Read the model definition and answer for the solid it produces. Units are mm, in the model's axes. A direction names the side the tool comes from. Give positions to 0.01 mm unless a question says otherwise; leave off trailing zeros. Loops run counter-clockwise (first coordinate to the right, second up) from the corner with the lowest first, then second, coordinate; pieces in that order, holes last. Notation, with made-up numbers: (32.25, -12) -> (71.25, -12) arc R23 ccw to (71.25, 24) -> close; hole circle Ø8 at (52, 43). An arc over 180 degrees is marked (long way). Write each question's results on one line, items separated by ' | '. Start each with the question number.
Item 1: Each of these flat-tipped pins is pushed along its axis until it touches: P1, Ø2.5, axis at x = 17.5, z = 3.5, coming from the +Y side; P2, Ø1, axis at x = 23.5, z = 3, coming from the -Y side; P3, Ø4, axis at y = 5, z = 4.5, coming from the +X side. Where does it stop, or does it pass through?
Item 2: Which of the six approach directions +Z, -Z, +X, -X, +Y, -Y give full straight-line access (tool end or side, diameter ignored) to faces 4 (the flat face through (5, 15, 0)), 5 (the flat face through (20, 12.5, 5)), 6 (the flat face through (10, 24, 6))?
Item 3: Section A-A on y = 25 is taken. Write down the section's boundary in (x, z).
Item 4: Section B-B on z = 4.5 is taken. Write down the section's boundary in (x, y), and give its area (3 significant figures).
Item 5: Section D-D on z = 2.5 is taken. Write down the section's boundary in (x, y).
Item 6: Section C-C on x = 3 is taken. Write down the section's boundary in (y, z), and give its area (3 significant figures).
Item 7: Determine the mould class of faces 1 (the conical face through (19.965, 13.768, 7.393)), 2 (the flat face through (0, 15, 5)), 3 (the cylindrical face through (5, 5, 6)) for opening direction X: +X half, -X half, draft (parallel to the pull), parting line (faces both ways), or undercut.
Item 8: Find the intervals of material crossed by line 1 (Y direction, x = 3.25, z = 4.5); line 2 (Y direction, x = 3.5, z = 3.25); line 3 (Z direction, x = 5.25, y = 5), in increasing order.
```python
from build123d import *

# Parameters (mm, degrees)
SKETCH1_W           = 10
SKETCH1_H           = 9
BOSS_EXTRUDE1_DEPTH = 30
SKETCH2_W           = 9
SKETCH2_H           = 5
BOSS_EXTRUDE2_DEPTH = 20
SKETCH3_R           = 1.5
CUT_EXTRUDE1_DEPTH  = 38.161808352


# Read off the part's stored shape, not the designer's step: Cut-Extrude2
with BuildPart() as part:
    # Sketch1 → Boss-Extrude1 (new body)
    with BuildSketch(Plane(origin=(0, 0, 0), x_dir=(1, 0, 0), z_dir=(0, 1, 0))):
        with Locations((5, -4.5)):
            Rectangle(SKETCH1_W, SKETCH1_H)
    extrude(amount=BOSS_EXTRUDE1_DEPTH)

    # Sketch2 → Boss-Extrude2 (add)
    with BuildSketch(Plane(origin=(10, 0, 0), x_dir=(0, 0, -1), z_dir=(1, 0, 0))):
        with Locations((-4.5, 15)):
            Rectangle(SKETCH2_W, SKETCH2_H)
    extrude(amount=BOSS_EXTRUDE2_DEPTH)

    # Sketch3 → Cut-Extrude1 (cut, through all)
    with BuildSketch(Plane(origin=(10, 0, 0), x_dir=(0, 0, -1), z_dir=(1, 0, 0))):
        with Locations((-4.5, 25)):
            Circle(SKETCH3_R)
        with Locations(Location((-4.5, 5, 0), (0, 0, 180))):
            Circle(SKETCH3_R)
    extrude(amount=-CUT_EXTRUDE1_DEPTH, mode=Mode.SUBTRACT)

    # Cut-Extrude2 outline → Cut-Extrude2 (revolve, cut)
    with BuildSketch(Plane(origin=(20, 0, 0), x_dir=(1, 0, 0), z_dir=(0, 0, 1))):
        Polygon((1.718721659, 12.5), (1.5, 15), (1.718721659, 17.5), (0, 17.5), (0, 12.5), align=None)
    cut_extrude2 = revolve(axis=Axis((20, 0, 0), (0, 1, 0)), mode=Mode.SUBTRACT)

    # Mirror1: Cut-Extrude2 across plane
    add(cut_extrude2.mirror(Plane.XY.offset(4.5)), mode=Mode.SUBTRACT)


solid = part.part
```
Findings:
1) P1: y = 17.5 | P2: y = 12.5 | P3: x = 10
2) face 4: -Z, +X, -X, +Y, -Y | face 5: +Z, -Z, +X, -Y | face 6: +Z, -Z, +X, +Y
3) outline: (0, 0) -> (10, 0) -> (10, 3) -> (0, 3) -> close; (0, 6) -> (10, 6) -> (10, 9) -> (0, 9) -> close
4) outline: (0, 0) -> (10, 0) -> (10, 3.5) -> (0, 3.5) -> close; (0, 6.5) -> (10, 6.5) -> (10, 12.5) -> (30, 12.5) -> (30, 17.5) -> (10, 17.5) -> (10, 23.5) -> (0, 23.5) -> close; (0, 26.5) -> (10, 26.5) -> (10, 30) -> (0, 30) -> close | area: 340 mm2
5) outline: (0, 0) -> (10, 0) -> (10, 12.5) -> (30, 12.5) -> (30, 17.5) -> (10, 17.5) -> (10, 30) -> (0, 30) -> close
6) outline: (0, 0) -> (30, 0) -> (30, 9) -> (0, 9) -> close; hole circle Ø3 at (5, 4.5); hole circle Ø3 at (25, 4.5) | area: 256 mm2
7) face 1: undercut | face 2: -X half | face 3: draft
8) line 1: 0 to 3.5, 6.5 to 23.5, 26.5 to 30 | line 2: 0 to 4.17, 5.83 to 24.17, 25.83 to 30 | line 3: 0 to 3, 6 to 9
